For this review, take the finished solid that the model builds, in its own axes (mm). Face numbers are marked on the shaded views. A direction names the side the tool comes from. Coordinates: 2 decimals unless noted, no trailing zeros. Loops run counter-clockwise (first coordinate to the right, second up) from the corner with the lowest first, then second, coordinate; pieces in that order, holes last. Notation, with made-up numbers: (70.25, -2.75) -> (82.25, -2.75) arc R22 cw to (82.25, 31.25) -> close; hole circle Ø6 at (47, -5). An arc over 180 degrees is marked (long way). One line per item, written item: value.
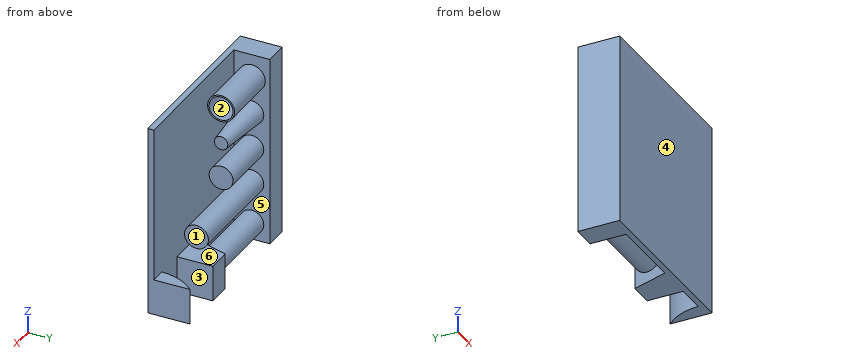
from build123d import *

# Parameters (mm, degrees)
BOSS_EXTRUDE1_DEPTH             = 640
BOSS_EXTRUDE2_DEPTH             = 120
ONE_SIDE_R                      = 40
BOSS_EXTRUDE4_DEPTH             = 251.6
BOTH_SIDES_R                    = 40
BOSS_EXTRUDE5_DEPTH             = 200
BOSS_EXTRUDE5_DIRECTION_2_REACH = 242
SOLID_2_R                       = 40
BOSS_EXTRUDE6_DEPTH             = 200
DRAFT_2_R                       = 40
BOSS_EXTRUDE7_DEPTH             = 200
BOSS_EXTRUDE7_TAPER             = 5
THICKEN_2_R                     = 45
THICKEN_2_R_2                   = 40
EXTRUDE_THIN1_DEPTH             = 200


with BuildPart() as part:
    # Sketch1 → Boss-Extrude1 (new body)
    with BuildSketch(Plane.XY):
        Polygon((-300, 0), (300, 0), (300, 20), (-220, 20), (-220, 140), (-300, 140), align=None)
    extrude(amount=BOSS_EXTRUDE1_DEPTH)

    # Sketch2 → Boss-Extrude2 (add)
    with BuildSketch(Plane.XY):
        with BuildLine():
            Line((300, 140), (300, 20))
            Line((300, 20), (247.956312481, 20))
            ThreePointArc((247.956312481, 20), (262.414199332, 85.015257999), (300, 140))
        make_face()
        Polygon((150, 140), (70, 140), (31.6, 20), (150, 20), align=None)
    extrude(amount=BOSS_EXTRUDE2_DEPTH)

    # One_Side → Boss-Extrude4 (add)
    with BuildSketch(Plane(origin=(-220, 0, 0), x_dir=(0, 0, -1), z_dir=(1, 0, 0))):
        with Locations((-60, 80)):
            Circle(ONE_SIDE_R)
    extrude(amount=BOSS_EXTRUDE4_DEPTH)

    # Both_Sides → Boss-Extrude5 (add)
    with BuildSketch(Plane(origin=(-60, 0, 0), x_dir=(0, 0, -1), z_dir=(1, 0, 0))):
        with Locations((-200, 80)):
            Circle(BOTH_SIDES_R)
    extrude(amount=BOSS_EXTRUDE5_DEPTH)

    # Both_Sides → Boss-Extrude5 direction 2 (add, up to next)
    with BuildSketch(Plane(origin=(-60, 0, 0), x_dir=(0, 0, -1), z_dir=(1, 0, 0)), mode=Mode.PRIVATE) as boss_extrude5_direction_2_sk1:
        with Locations((-200, 80)):
            Circle(BOTH_SIDES_R)
    boss_extrude5_direction_2_tool1 = extrude(boss_extrude5_direction_2_sk1.sketch, amount=-BOSS_EXTRUDE5_DIRECTION_2_REACH, mode=Mode.PRIVATE) - part.part
    add(boss_extrude5_direction_2_tool1.solids().sort_by_distance((-60, 80, 200))[0])

    # Solid 2 → Boss-Extrude6 (add)
    with BuildSketch(Plane(origin=(-220, 0, 0), x_dir=(0, 0, -1), z_dir=(1, 0, 0))):
        with Locations((-320, 80)):
            Circle(SOLID_2_R)
    extrude(amount=BOSS_EXTRUDE6_DEPTH)

    # Draft 2 → Boss-Extrude7 (add)
    with BuildSketch(Plane(origin=(-220, 0, 0), x_dir=(0, 0, -1), z_dir=(1, 0, 0))):
        with Locations((-440, 80)):
            Circle(DRAFT_2_R)
    extrude(amount=BOSS_EXTRUDE7_DEPTH, taper=BOSS_EXTRUDE7_TAPER)

    # Thicken 2 → Extrude-Thin1 (add)
    with BuildSketch(Plane(origin=(-220, 0, 0), x_dir=(0, 0, -1), z_dir=(1, 0, 0))):
        with Locations((-560, 80)):
            Circle(THICKEN_2_R)
        with Locations((-560, 80)):
            Circle(THICKEN_2_R_2, mode=Mode.SUBTRACT)
    extrude(amount=EXTRUDE_THIN1_DEPTH)


solid = part.part
1. Insertion check: pin 1 Ø10 at (y, z) = (45.5, 365.5) entering from +X; pin 2 Ø24 at (y, z) = (80.5, 181.5) entering from +X; pin 3 Ø10 at (x, y) = (5.5, 62.5) entering from +Z. Each pin has a flat end and moves straight along its axis. Give the tip position at first contact, or say it passes through.
Return value:
pin 1: stops at x = -220
pin 2: stops at x = 140
pin 3: stops at z = 238
2. To check wall thickness, follow probe 1 along Y at (x, z) = (-88, 560); probe 2 along Z at (x, y) = (-161.5, 89); probe 3 along X at (y, z) = (123, 78.5). State the ranges of each line that lie inside material, in increasing order. Write a range as from..to.
Return value:
probe 1: y = 0..20, 35..40, 120..125
probe 2: z = 21.03..98.97, 161.03..238.97, 281.03..358.97, 406.3..473.7, 515.91..521.03, 598.97..604.09
probe 3: x = -300..-220, 64.56..150, 284.93..300
3. For the marked faces 1, 2 and 3, list the 3-axis set-ups (+Z, -Z, +X, -X, +Y, -Y) from which the entire face can be reached by the end or side of a thin tool; tool diameter is ignored.
Return value:
face 1: +Z, +X, +Y
face 2: +X
face 3: +Z, -Z, +Y
4. Take a section at D-D, the plane z = 560. Give the boundary of the cut face in (x, y).
Return value:
outline: (-300, 0) -> (300, 0) -> (300, 20) -> (-220, 20) -> (-220, 35) -> (-20, 35) -> (-20, 40) -> (-220, 40) -> (-220, 120) -> (-20, 120) -> (-20, 125) -> (-220, 125) -> (-220, 140) -> (-300, 140) -> close
5. Take a section at B-B, the plane z = 440. Give the boundary of the cut face in (x, y).
Return value:
outline: (-300, 0) -> (300, 0) -> (300, 20) -> (-220, 20) -> (-220, 40) -> (-20, 57.5) -> (-20, 102.5) -> (-220, 120) -> (-220, 140) -> (-300, 140) -> close
6. Take a section at A-A, the plane x = -113.5. Give the boundary of the cut face in (y, z).
Return value:
outline: (0, 0) -> (20, 0) -> (20, 640) -> (0, 640) -> close; circle Ø90 at (80, 560); circle Ø80 at (80, 60); circle Ø80 at (80, 200); circle Ø80 at (80, 320); circle Ø61.36 at (80, 440); hole circle Ø80 at (80, 560)
7. The part is to be moulded in two halves that separate along Y. For the marked faces 4, 5 and 6, say which applies: pulls with the +Y half, pulls with the -Y half, needs draft (parallel to the pull), parting line crosses it, or undercut.
Return value:
face 4: pulls with the -Y half
face 5: undercut
face 6: needs draft
8. Take a section at C-C, the plane y = 80. Give the number of separate pieces and of enclosed holes in the cut face, and give its area (3 significant figures).
Return value:
separate pieces: 3
enclosed holes: 0
area: 147,000 mm2
